from build123d import *

# Parameters (mm, degrees)
F0_W     = 25.4
F0_H     = 25.4
F0_W_2   = 22.86
F0_H_2   = 22.86
F1_DEPTH = 228.6
F2_R     = 5.08


with BuildPart() as f1:
    # F0 (on Front) → F1 (new body, symmetric)
    with BuildSketch(Plane.XZ):
        Rectangle(F0_W, F0_H)
        Rectangle(F0_W_2, F0_H_2, mode=Mode.SUBTRACT)
    extrude(amount=F1_DEPTH, both=True)

    # F2
    f2_edges = [f1.edges().sort_by_distance(p)[0] for p in [
        (-11.43, 0, 11.43),
        (11.43, 0, 11.43),
        (-11.43, 0, -11.43),
        (11.43, 0, -11.43),
        (-12.7, 0, 12.7),
        (12.7, 0, 12.7),
        (-12.7, 0, -12.7),
        (12.7, 0, -12.7),
    ]]
    fillet(f2_edges, radius=F2_R)


solid = f1.part
Model file for the job. Use its own axes, mm. A direction names the side the tool comes from. Give positions to 0.01 mm unless a question says otherwise; leave off trailing zeros. Order: outer loops, then holes, each group sorted by start corner. A loop starts at its lowest first (then second) coordinate and runs counter-clockwise, first axis right, second up. Notation, with made-up numbers: (8, 76.5) - (23, 76.5) arc R31 cw to (23, 112.5) - close; hole circle Ø9 at (-16.5, 50.25). An arc over 180 degrees is marked (long way). Return JSON: item names as keys, results as strings.
1) 3-axis set-ups, long thin cutter, end or side, ignore diameter. For faces 1 (the flat face through (-12.7, -3, 0)), 2 (the flat face through (11.43, -3, 0)): which of +Z, -Z, +X, -X, +Y, -Y reach the whole face in a straight line?
Geometry says:
{"face 1": "+Z, -Z, -X, +Y, -Y", "face 2": "+Y, -Y"}
2) Probe line 1 (Z direction, x = 4, y = -142); line 2 (Z direction, x = 9, y = 89). List the from-to ranges inside material, lowest first. Write a range as from..to.
Geometry says:
{"line 1": "-12.7..-11.43, 11.43..12.7", "line 2": "-12.51..-10.68, 10.68..12.51"}
3) Pull direction X, two halves, no side cores. Call faces 3 (the flat face through (0, -3, -11.43)), 4 (the flat face through (0, -3, -12.7)), 5 (the flat face through (12.7, -3, 0)): pulls with the +X half, pulls with the -X half, needs draft (parallel to the pull), parting line crosses it, or undercut.
Geometry says:
{"face 3": "undercut", "face 4": "needs draft", "face 5": "pulls with the +X half"}
4) Cut at A-A, the plane y = -44. Give the cut face in (x, z), plus the area to 3 significant figures.
Geometry says:
{"outline": "(-12.7, -7.62) arc R5.08 ccw to (-7.62, -12.7) - (7.62, -12.7) arc R5.08 ccw to (12.7, -7.62) - (12.7, 7.62) arc R5.08 ccw to (7.62, 12.7) - (-7.62, 12.7) arc R5.08 ccw to (-12.7, 7.62) - close; hole (-11.43, -6.35) arc R5.08 ccw to (-6.35, -11.43) - (6.35, -11.43) arc R5.08 ccw to (11.43, -6.35) - (11.43, 6.35) arc R5.08 ccw to (6.35, 11.43) - (-6.35, 11.43) arc R5.08 ccw to (-11.43, 6.35) - close", "area": "123 mm²"}
5) Cut at B-B, the plane x = -2.25. Give the cut face in (y, z), plus the area to 3 significant figures.
Geometry says:
{"outline": "(-228.6, -12.7) - (228.6, -12.7) - (228.6, -11.43) - (-228.6, -11.43) - close; (-228.6, 11.43) - (228.6, 11.43) - (228.6, 12.7) - (-228.6, 12.7) - close", "area": "1,160 mm²"}
